Input: part model. Units: mm. Frame: model coordinates. A direction names the side the tool comes from. Round coordinates to 2 decimals unless told otherwise and drop trailing zeros. Loops run counter-clockwise (first coordinate to the right, second up) from the corner with the lowest first, then second, coordinate; pieces in that order, holes last. Notation, with made-up numbers: (30, -11.75) - (82, -11.75) arc R11 ccw to (82, 3.25) - close; hole circle Ø2 at (63, 11.25). An arc over 180 degrees is marked (long way). Use CSV: the item, a comma, the result in double quotes. Start each with the question number.
1. Cut plane D-D (y = 0.5). Return loops of the section in (x, z).
2. Cut plane C-C (y = -3.5). Return loops of the section in (x, z).
3. Cut plane A-A (z = 0). Return loops of the section in (x, y), and give its area (3 significant figures).
4. Pin query (flat end, axial travel): P1, Ø3, axis at x = -1, y = -3.5, coming from the +Z side; P2, Ø1, axis at x = -0.5, z = -2, coming from the -Y side; P3, Ø4, axis at y = 0, z = -2, coming from the +X side; P4, Ø1, axis at x = -0.5, y = -1.5, coming from the -Z side. Return the tip coordinate at first contact, or that it passes through.
5. Access query for faces 1 (the cylindrical face through (-3.955, 1.479, -5.158)), 2 (the cylindrical face through (0.45, -2.71, 1.43)). Directions: +Z, -Z, +X, -X, +Y, -Y. A direction counts if a zero-diameter tool reaches every point of the face in a straight line with its end or side. Return the directions, or none.
6. Cut plane B-B (x = 0). Return loops of the section in (y, z).
7. Material intervals for probe 1 along Y at (x, z) = (4.75, -2.5); probe 2 along Z at (x, y) = (5.25, 1.5); probe 3 along X at (y, z) = (-0.75, 0), sorted ascending. Write a range as from..to.
```python
from build123d import *

# Parameters (mm, degrees)
SKETCH1_R           = 6.5
BOSS_EXTRUDE1_DEPTH = 3
SKETCH2_R           = 1.5
BOSS_EXTRUDE2_DEPTH = 6
FILLET1_R           = 0.5


with BuildPart() as part:
    # Sketch1 → Boss-Extrude1 (new body)
    with BuildSketch(Plane(origin=(0, 0, 0), x_dir=(1, 0, 0), z_dir=(0, 1, 0))):
        with Locations(Location((0, 0, 0), (0, 0, 270))):
            Circle(SKETCH1_R)
    extrude(amount=BOSS_EXTRUDE1_DEPTH)

    # Sketch2 → Boss-Extrude2 (add)
    with BuildSketch(Plane(origin=(0, 0, 0), x_dir=(1, 0, 0), z_dir=(0, 1, 0))):
        with Locations(Location((0, 0, 0), (0, 0, 270))):
            Circle(SKETCH2_R)
    extrude(amount=-BOSS_EXTRUDE2_DEPTH)

    # Fillet1
    fillet1_edges = [part.edges().sort_by_distance(p)[0] for p in [
        (0, -6, -1.5),
    ]]
    fillet(fillet1_edges, radius=FILLET1_R)


solid = part.part
```
Established:
1,outline,"circle Ø13 at (0, 0)"
2,outline,"circle Ø3 at (0, 0)"
3,outline,"(-6.5, 0) - (-1.5, 0) - (-1.5, -5.5) arc R0.5 ccw to (-1, -6) - (1, -6) arc R0.5 ccw to (1.5, -5.5) - (1.5, 0) - (6.5, 0) - (6.5, 3) - (-6.5, 3) - close"
3,area,"56.9 mm2"
4,P1,"stops at z = 1.5"
4,P2,"stops at y = 0"
4,P3,"stops at x = 6.5"
4,P4,"stops at z = -1.5"
5,face 1,"+Y, -Y"
5,face 2,"-Y"
6,outline,"(-6, -1) arc R0.5 ccw to (-5.5, -1.5) - (0, -1.5) - (0, -6.5) - (3, -6.5) - (3, 6.5) - (0, 6.5) - (0, 1.5) - (-5.5, 1.5) arc R0.5 ccw to (-6, 1) - close"
7,probe 1,"y = 0..3"
7,probe 2,"z = -3.83..3.83"
7,probe 3,"x = -1.5..1.5"
